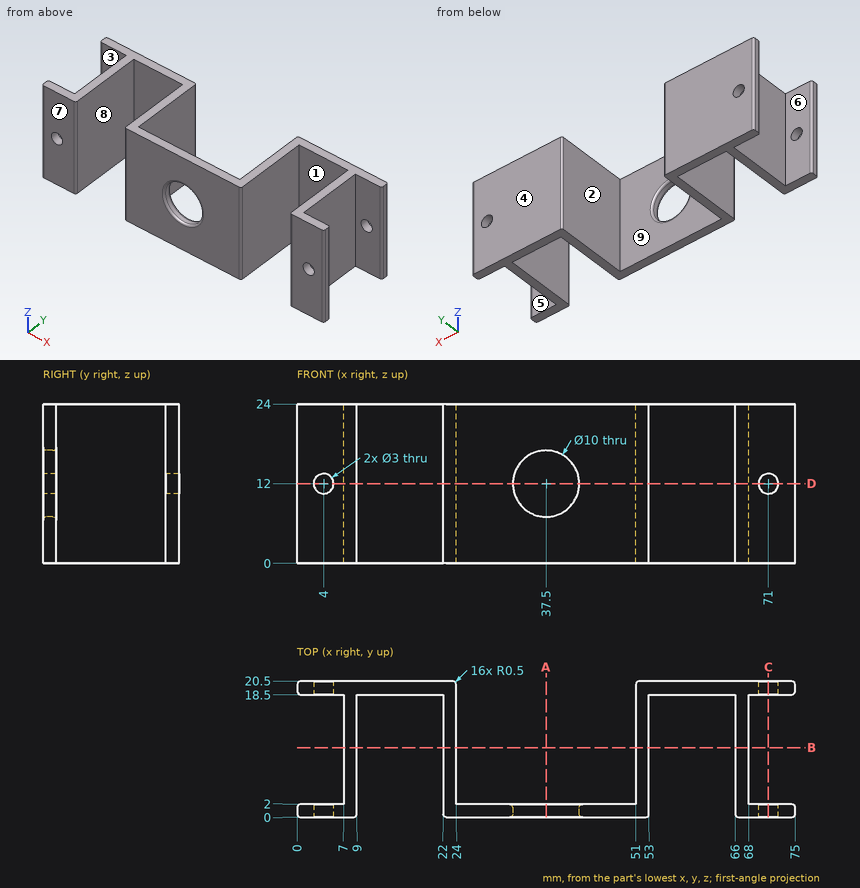
Print and shaded views of the part. All mm, measured from the part's lowest x, y and z. A direction names the side the tool comes from. Give positions to 0.01 mm unless a question says otherwise; leave off trailing zeros. Write each loop counter-clockwise with the first axis right and the second up, starting at its lowest first coordinate (ties: lowest second). Pieces come first, ordered by that corner, then holes. Notation, with made-up numbers: (77.5, 4) - (126.5, 4) arc R16 ccw to (126.5, 11) - close; hole circle Ø7 at (9.25, 47.25). An arc over 180 degrees is marked (long way). Put each result on its own line as item: value.
(1) Saw through at A-A (x = 37.5). List the corners of the cut face in (y, z).
Working result:
outline: (0, 0) - (2, 0) - (2, 6.5) arc R0.5 ccw to (1.5, 7) - (0.5, 7) arc R0.5 ccw to (0, 6.5) - close; (0, 17.5) arc R0.5 ccw to (0.5, 17) - (1.5, 17) arc R0.5 ccw to (2, 17.5) - (2, 24) - (0, 24) - close
(2) Wall check: L1, parallel to X at y = 2.25, z = 11; L2, parallel to Z at x = 71, y = 0.9; L3, parallel to Y at x = 19.5, z = 17.25. Give the ranges that are in metal, low to high.
Working result:
L1: 7 to 9, 22 to 24, 51 to 53, 66 to 68
L2: 0 to 10.5, 13.5 to 24
L3: 18.5 to 20.5
(3) Saw through at B-B (y = 10.5). List the corners of the cut face in (x, z).
Working result:
outline: (7, 0) - (9, 0) - (9, 24) - (7, 24) - close; (22, 0) - (24, 0) - (24, 24) - (22, 24) - close; (51, 0) - (53, 0) - (53, 24) - (51, 24) - close; (66, 0) - (68, 0) - (68, 24) - (66, 24) - close
(4) Pull direction Y, two halves, no side cores. Call the marked faces 6, 7, 8 and 9: released by +Y, released by -Y, zero draft, split by the parting line, or undercut.
Working result:
face 6: undercut
face 7: released by -Y
face 8: zero draft
face 9: released by +Y
(5) Drop flat-ended pins along their axis: pin 1 Ø10.5 at (x, z) = (59.5, 10) entering from -Y; pin 2 Ø8 at (y, z) = (10.5, 11.5) entering from -X; pin 3 Ø12 at (y, z) = (8.5, 17.5) entering from +X. Give the stop position or say it passes through.
Working result:
pin 1: y = 18.5
pin 2: x = 7
pin 3: x = 68
(6) Tool access for the marked faces 1, 2, 3, 4 and 5: list every direction of +Z, -Z, +X, -X, +Y, -Y with a clear straight run to the whole face (end or side of a thin tool).
Working result:
face 1: +Z, -Z, -Y
face 2: +Z, -Z, +Y
face 3: +Z, -Z, -X
face 4: +Z, -Z, +X, -X, +Y
face 5: +Z, -Z, +X
(7) Saw through at C-C (x = 71). List the corners of the cut face in (y, z).
Working result:
outline: (0, 0) - (2, 0) - (2, 10.5) - (0, 10.5) - close; (0, 13.5) - (2, 13.5) - (2, 24) - (0, 24) - close; (18.5, 0) - (20.5, 0) - (20.5, 10.5) - (18.5, 10.5) - close; (18.5, 13.5) - (20.5, 13.5) - (20.5, 24) - (18.5, 24) - close
(8) Saw through at D-D (z = 12). Count the separate pieces of the cut face and the enclosed holes in it, then the cut area to 3 significant figures.
Working result:
separate pieces: 6
enclosed holes: 0
area: 281 mm^2
